```python
from build123d import *

# Parameters (mm, degrees)
SKETCH1_W           = 63.335064935
SKETCH1_H           = 65.606575703
BOSS_EXTRUDE1_DEPTH = 50
CUT_EXTRUDE1_DEPTH  = 50
CUT_EXTRUDE2_REACH  = 80.83
SKETCH3_R           = 8.5


with BuildPart() as part:
    # Sketch1 → Boss-Extrude1 (new body)
    with BuildSketch(Plane.XY):
        with Locations((31.667532468, 32.803287852)):
            Rectangle(SKETCH1_W, SKETCH1_H)
    extrude(amount=BOSS_EXTRUDE1_DEPTH)

    # Sketch2 → Cut-Extrude1 (cut)
    with BuildSketch(Plane.XY.offset(50)):
        Polygon((25.457090792, 65.606575703), (63.335064935, 0), (63.335064935, 65.606575703), align=None)
    extrude(amount=-CUT_EXTRUDE1_DEPTH, mode=Mode.SUBTRACT)

    # Cut-Extrude2: up to this plane
    cut_extrude2_end = Plane(origin=(0, 0, 50), z_dir=(-1, 0, 0))
    # Sketch3 → Cut-Extrude2 (cut, up to the surface)
    with BuildSketch(Plane(origin=(47.501298701, 27.424887592, 0), x_dir=(0, 0, -1), z_dir=(0.866025403784436, 0.5000000000000043, 0)), mode=Mode.PRIVATE) as cut_extrude2_sk1:
        with Locations(Location((-25, 22.143442983, 0), (0, 0, 90))):
            Circle(SKETCH3_R)
    cut_extrude2_tool1 = split(extrude(cut_extrude2_sk1.sketch, amount=-CUT_EXTRUDE2_REACH, mode=Mode.PRIVATE), bisect_by=cut_extrude2_end, keep=Keep.BOTH, mode=Mode.PRIVATE)
    add(cut_extrude2_tool1.solids().sort_by_distance((36.429577, 46.601672, 25))[0], mode=Mode.SUBTRACT)


solid = part.part
```
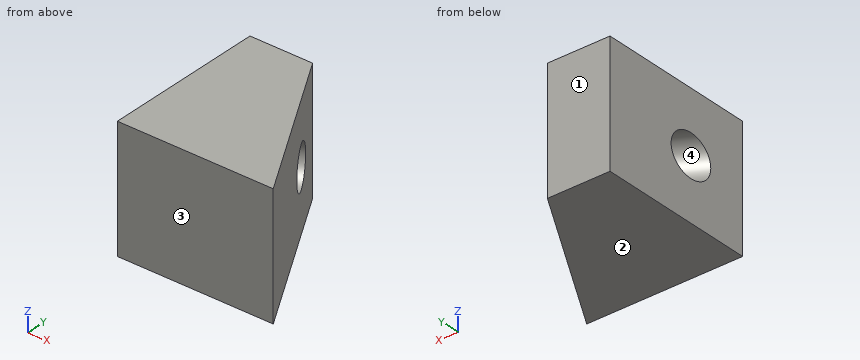
CAD build for the part. Positions are in the model's coordinates, mm. Face numbers are marked on the shaded views. Round coordinates to 2 decimals unless told otherwise and drop trailing zeros. Order: outer loops, then holes, each group sorted by start corner. A loop starts at its lowest first (then second) coordinate and runs counter-clockwise, first axis right, second up.
Q1. Slice it at C-C (y = 6.5). Write the cut outline in (x, z), and give its area (3 significant figures).
Q2. Slice it at A-A (z = 23). Write the cut outline in (x, y).
Q3. Drop flat-ended pins along their axis: pin 1 (2 mm diameter, centred on y = 36, z = 13.5, fed in from +X); pin 2 (12 mm diameter, centred on y = 47, z = 35.5, fed in from +X); pin 3 (3 mm diameter, centred on x = 49.5, y = 29, fed in from -Z); pin 4 (8 mm diameter, centred on y = 12.5, z = 44, fed in from +X). Give the stop position or say it passes through.
Q4. Two-plate mould, pull along Y, no slides. Class the marked faces 1, 2, 3 and 4: pulls with the +Y half, pulls with the -Y half, needs draft (parallel to the pull), parting line crosses it, or undercut.
Q5. Wall check: L1, parallel to Z at x = 13.5, y = 33.5; L2, parallel to X at y = 36, z = 22.5; L3, parallel to Y at x = 3, z = 25.5. Give the ranges that are in metal, low to high.
Q6. Slice it at B-B (z = 40.5). Write the cut outline in (x, y), and give its area (3 significant figures).
Results below:
1. outline: (0, 0) - (59.58, 0) - (59.58, 50) - (0, 50) - close
1. area: 2,980 mm2
2. outline: (0, 0) - (63.34, 0) - (40.56, 39.45) - (0, 16.03) - close; (0, 35.11) - (32.3, 53.76) - (25.46, 65.61) - (0, 65.61) - close
3. pin 1: stops at x = 43.13
3. pin 2: stops at x = 39.66
3. pin 3: passes through
3. pin 4: stops at x = 58.43
4. face 1: pulls with the +Y half
4. face 2: needs draft
4. face 3: pulls with the -Y half
4. face 4: undercut
5. L1: z = 0 to 16.5, 33.5 to 50
5. L2: x = 0 to 1.82, 34.32 to 42.55
5. L3: y = 0 to 17.5, 37.1 to 65.61
6. outline: (0, 0) - (63.34, 0) - (25.46, 65.61) - (0, 65.61) - close
6. area: 2,910 mm2
